Job drawing, mm, ordinate dimensions from the low corner. One solid piece. A direction names the side the tool comes from. Give positions to 0.01 mm unless a question says otherwise; leave off trailing zeros. Write each loop counter-clockwise with the first axis right and the second up, starting at its lowest first coordinate (ties: lowest second). Pieces come first, ordered by that corner, then holes. Notation, with made-up numbers: M -35,81.5 L -21,81.5 A24 ccw -21,91.5 Z; hole C 12,28.5 d6. An arc over 180 degrees is marked long. Use a Markdown table: item, result.
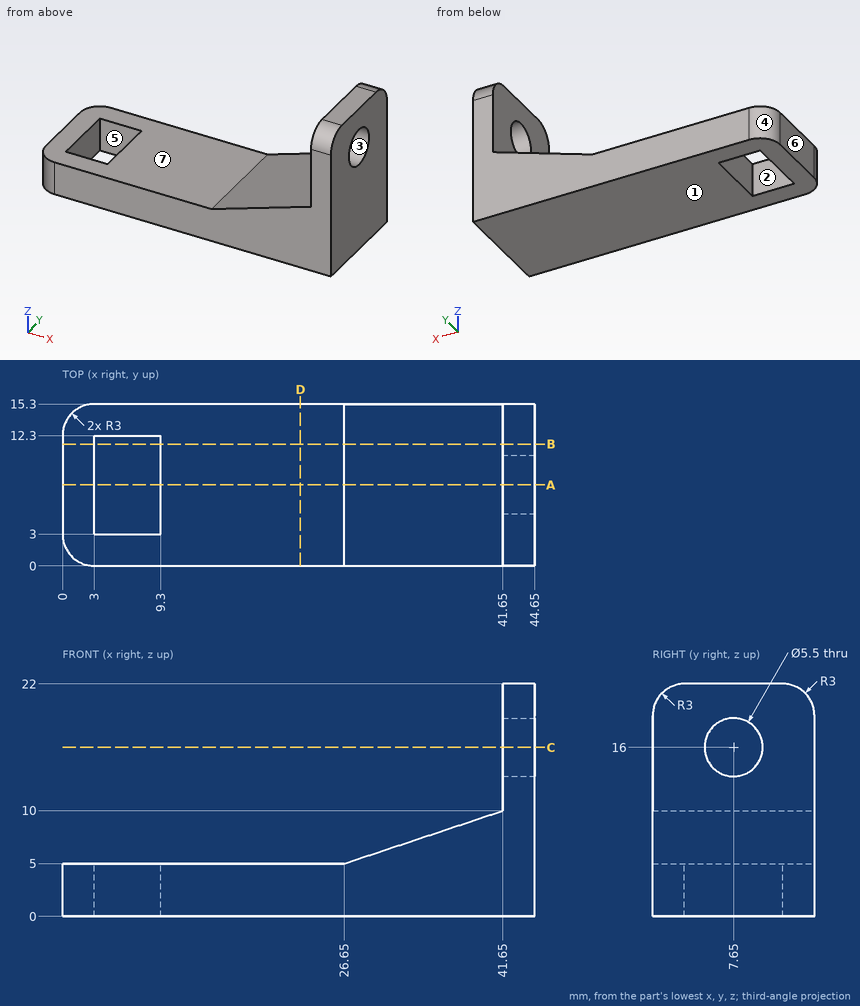
1. Two-plate mould, pull along Y, no slides. Class the marked faces 1, 2, 3 and 4: released by +Y, released by -Y, zero draft, split by the parting line, or undercut.
Findings below:
| item | result |
|---|---|
| face 1 | zero draft |
| face 2 | undercut |
| face 3 | undercut |
| face 4 | released by +Y |
2. Drill centre lines: L1, parallel to X at y = 7.5, z = 3.25; L2, parallel to Z at x = 42.4, y = 7.65; L3, parallel to Y at x = 43.4, z = 16. Where is each one in solid material? Low to high.
Findings below:
| item | result |
|---|---|
| L1 | 0 to 3, 9.3 to 44.65 |
| L2 | 0 to 13.25, 18.75 to 22 |
| L3 | 0 to 4.9, 10.4 to 15.3 |
3. Drop flat-ended pins along their axis: P1, Ø4.5, axis at y = 7.65, z = 16, coming from the -X side; P2, Ø4.5, axis at x = 12.5, y = 5, coming from the +Z side. Give the stop position or say it passes through.
Findings below:
| item | result |
|---|---|
| P1 | through |
| P2 | z = 5 |
4. Cut at C-C, the plane z = 16. Give the cut face in (x, y), then the cut area to 3 significant figures.
Findings below:
| item | result |
|---|---|
| outline | M 41.65,0 L 44.65,0 L 44.65,4.9 L 41.65,4.9 Z; M 41.65,10.4 L 44.65,10.4 L 44.65,15.3 L 41.65,15.3 Z |
| area | 29.4 mm2 |
5. Cut at A-A, the plane y = 7.65. Give the cut face in (x, z).
Findings below:
| item | result |
|---|---|
| outline | M 0,0 L 3,0 L 3,5 L 0,5 Z; M 9.3,0 L 44.65,0 L 44.65,13.25 L 41.65,13.25 L 41.65,10 L 26.65,5 L 9.3,5 Z; M 41.65,18.75 L 44.65,18.75 L 44.65,22 L 41.65,22 Z |
6. Cut at D-D, the plane x = 22.5. Give the cut face in (y, z), then the cut area to 3 significant figures.
Findings below:
| item | result |
|---|---|
| outline | M 0,0 L 15.3,0 L 15.3,5 L 0,5 Z |
| area | 76.5 mm2 |
7. Cut at B-B, the plane y = 11.5. Give the cut face in (x, z), then the cut area to 3 significant figures.
Findings below:
| item | result |
|---|---|
| outline | M 0,0 L 3,0 L 3,5 L 0,5 Z; M 9.3,0 L 44.65,0 L 44.65,22 L 41.65,22 L 41.65,10 L 26.65,5 L 9.3,5 Z |
| area | 280 mm2 |
8. Tool access for the marked faces 5, 6 and 7: list every direction of +Z, -Z, +X, -X, +Y, -Y with a clear straight run to the whole face (end or side of a thin tool).
Findings below:
| item | result |
|---|---|
| face 5 | +Z, -Z |
| face 6 | +Z, -Z, -X, +Y, -Y |
| face 7 | +Z, -X, +Y, -Y |
